For this review, use the dimensioned drawing (mm, ordinates from the lowest corner) and the shaded views. Coordinates: 2 decimals unless noted, no trailing zeros. Loops run counter-clockwise (first coordinate to the right, second up) from the corner with the lowest first, then second, coordinate; pieces in that order, holes last. Notation, with made-up numbers: (-40, 46) - (-21, 46) arc R20 cw to (-21, 71) - close; hole circle Ø5 at (64, 44). An arc over 180 degrees is marked (long way). One line per item, written item: value. Start each with the question number.
1. We need section B-B, the plane x = 17. Give the boundary of the cut face in (y, z), then the cut area to 3 significant figures.
2. To check wall thickness, follow line 1 (Y direction, x = 30, z = 0.8); line 2 (X direction, y = 4.25, z = 0.4); line 3 (X direction, y = 5.5, z = 0.15). State the ranges of each line that lie inside material, in increasing order.
3. Insertion check: P1, Ø0.6, axis at y = 5, z = 0.5, coming from the -X side. The pin has a flat end and moves straight along its axis. Give the tip position at first contact, or say it passes through.
4. We need section A-A, the plane z = 0.45. Give the boundary of the cut face in (x, y), then the cut area to 3 significant figures.
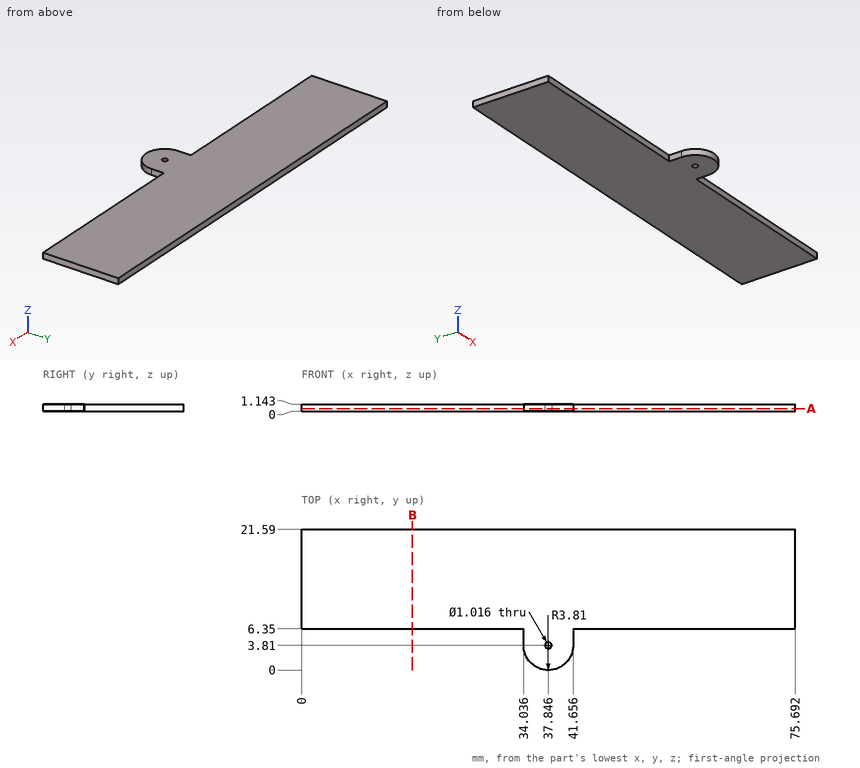
Findings below:
1. outline: (6.35, 0) - (21.59, 0) - (21.59, 1.14) - (6.35, 1.14) - close
1. area: 17.4 mm2
2. line 1: 6.35 to 21.59
2. line 2: 34.04 to 37.59, 38.1 to 41.66
2. line 3: 34.04 to 41.66
3. P1: x = 34.04
4. outline: (0, 6.35) - (34.04, 6.35) - (34.04, 3.81) arc R3.81 ccw to (41.66, 3.81) - (41.66, 6.35) - (75.69, 6.35) - (75.69, 21.59) - (0, 21.59) - close; hole circle Ø1.02 at (37.85, 3.81)
4. area: 1,190 mm2
